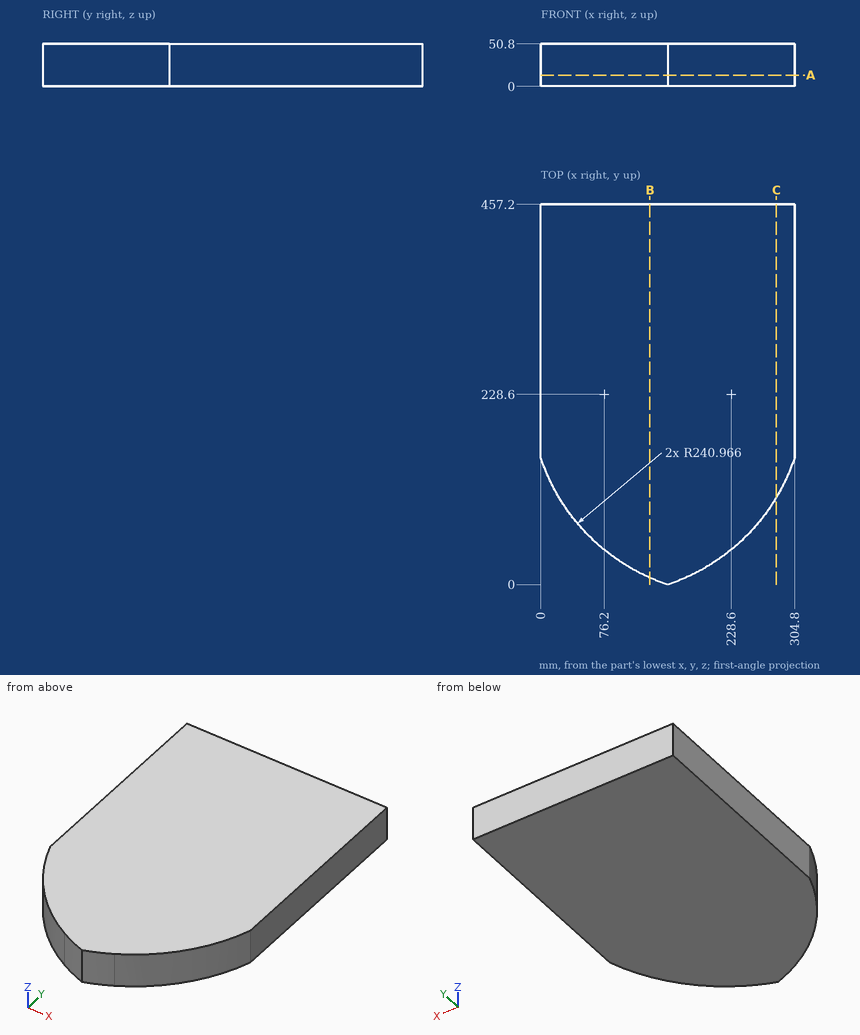
Verification items for this drawing (mm, ordinates from the low corner). Coordinates: 2 decimals unless noted, no trailing zeros. Loops run counter-clockwise (first coordinate to the right, second up) from the corner with the lowest first, then second, coordinate; pieces in that order, holes last. Notation, with made-up numbers: (-37, 28.5) -> (-13, 28.5) arc R20 cw to (-13, 66.5) -> close; hole circle Ø5 at (-19.75, 50). An arc over 180 degrees is marked (long way). Answer in a Markdown table with one row per item. Add a question column.
1. Material ranges on probe 1 along X at (y, z) = (25.5, 39) (1 decimal); probe 2 along X at (y, z) = (104, 29); probe 3 along Y at (x, z) = (104, 24), recorded low to high. Write a range as [from, to].
2. Depth check by flat-ended pin: P1, Ø3, axis at x = 129, z = 7.5, coming from the -Y side; P2, Ø2, axis at x = 134, z = 35, coming from the -Y side; P3, Ø2, axis at x = 175.5, z = 29, coming from the -Y side. Enter the tip coordinate at first touch or a pass-through.
3. Section check B-B, the plane x = 131. Enter the section's corners in (y, z) (1 decimal), then the cut area to 3 significant figures.
4. Section check C-C, the plane x = 283. Enter the section's corners in (y, z) (1 decimal), then the cut area to 3 significant figures.
5. Section check A-A, the plane z = 13.5. Enter the section's corners in (x, y) (1 decimal), then the cut area to 3 significant figures.
Derived:
| question | item | result |
|---|---|---|
| 1 | probe 1 | x = [98.9, 205.9] |
| 1 | probe 2 | x = [22.35, 282.45] |
| 1 | probe 3 | y = [22.35, 457.2] |
| 2 | P1 | stops at y = 8.51 |
| 2 | P2 | stops at y = 6.56 |
| 2 | P3 | stops at y = 8.6 |
| 3 | outline | (8.3, 0) -> (457.2, 0) -> (457.2, 50.8) -> (8.3, 50.8) -> close |
| 3 | area | 22,800 mm² |
| 4 | outline | (104.9, 0) -> (457.2, 0) -> (457.2, 50.8) -> (104.9, 50.8) -> close |
| 4 | area | 17,900 mm² |
| 5 | outline | (0, 152.4) arc R241 ccw to (152.4, 0) arc R241 ccw to (304.8, 152.4) -> (304.8, 457.2) -> (0, 457.2) -> close |
| 5 | area | 124,000 mm² |
